```python
from build123d import *

# Parameters (mm, degrees)
F1_DEPTH  = 600
F3_DEPTH  = 600.001
F5_DEPTH  = 20
F7_DEPTH  = 20
F8_W      = 20
F8_H      = 278.7190201738
F8_W_2    = 578.8190174103
F9_DEPTH  = 20
F10_W     = 598.5316634178
F10_H     = 254.7840774059
F11_DEPTH = 2017.6951884178


# Not quite as in the source:
# - a feature names something its author has since deleted; it is built from what else it names


with BuildPart() as f1:
    # F0 (on Right) → F1 (new body)
    with BuildSketch(Plane.YZ):
        with BuildLine():
            ThreePointArc((-413.7737442203, 1932.6941884178), (-235.6171133469, 874.7152717166), (-858.6646769196, 1.2904570733))
            Line((-858.6646769196, 1.2904570733), (841.3353230804, 1.2904570733))
            ThreePointArc((841.3353230804, 1.2904570733), (218.2877610308, 874.7152723164), (396.4443930804, 1932.6941884178))
            Line((396.4443930804, 1932.6941884178), (396.4443930804, 2017.6941884178))
            ThreePointArc((396.4443930804, 2017.6941884178), (199.7456261802, 1948.7680536266), (-8.6646769196, 1951.2904570733))
            ThreePointArc((-8.6646769196, 1951.2904570733), (-217.0749786293, 1948.7680541113), (-413.7737442203, 2017.6941884178))
            Line((-413.7737442203, 2017.6941884178), (-413.7737442203, 1932.6941884178))
        make_face()
    extrude(amount=F1_DEPTH)

    # F2 (on face) → F3 (cut, through all)
    with BuildSketch(Plane.YZ.offset(600)):
        with BuildLine():
            Line((396.4443930804, 2017.6941884178), (-413.7737442203, 2017.6941884178))
            ThreePointArc((-413.7737442203, 2017.6941884178), (-345.7057427079, 1986.5957603046), (-275.2746839195, 1961.3008790249))
            ThreePointArc((-275.2746839195, 1961.3008790249), (-142.5331399832, 1941.2889121961), (-8.6646769196, 1951.2904570733))
            ThreePointArc((-8.6646769196, 1951.2904570733), (125.2037851776, 1941.2889117025), (257.9453283126, 1961.3008776288))
            ThreePointArc((257.9453283126, 1961.3008776288), (328.3763894007, 1986.5957594221), (396.4443930804, 2017.6941884178))
        make_face()
        with BuildLine():
            ThreePointArc((-8.6646769196, 1951.2904570733), (-142.5331399832, 1941.2889121961), (-275.2746839195, 1961.3008790249))
            ThreePointArc((-275.2746839195, 1961.3008790249), (-8.66467791, 1920.6086514411), (257.9453283126, 1961.3008776288))
            ThreePointArc((257.9453283126, 1961.3008776288), (125.2037851776, 1941.2889117025), (-8.6646769196, 1951.2904570733))
        make_face()
    extrude(amount=-F3_DEPTH, mode=Mode.SUBTRACT)

    # F4 (on face) → F5 (join)
    with BuildSketch(Plane.YZ.offset(600)):
        with BuildLine():
            ThreePointArc((-487.8719790556, 1039.6971702576), (-533.5033840935, 470.5867589871), (-858.6646769196, 1.2904570733))
            ThreePointArc((-858.6646769196, 1.2904570733), (-413.6127871917, 445.5030116798), (-207.8719790556, 1039.6971702576))
            Line((-207.8719790556, 1039.6971702576), (-487.8719790556, 1039.6971702576))
        make_face()
        with BuildLine():
            ThreePointArc((190.5426270267, 1039.6971702576), (396.283434362, 445.5030119538), (841.3353230804, 1.2904570733))
            ThreePointArc((841.3353230804, 1.2904570733), (516.1740306428, 470.5867590462), (470.5426270267, 1039.6971702576))
            Line((470.5426270267, 1039.6971702576), (190.5426270267, 1039.6971702576))
        make_face()
    extrude(amount=-F5_DEPTH)

    # F6 (on face) → F7 (join)
    with BuildSketch(Plane(origin=(0, 0, 0), x_dir=(0, -1, 0), z_dir=(-1, 0, 0))):
        with BuildLine():
            ThreePointArc((-841.3353230804, 1.2904570733), (-396.5475396439, 445.0817710452), (-190.6490020093, 1038.7085012816))
            Line((-190.6490020093, 1038.7085012816), (-470.6490020093, 1038.7085012816))
            ThreePointArc((-470.6490020093, 1038.7085012816), (-519.6815928842, 471.2934981386), (-841.3353230804, 1.2904570733))
        make_face()
        with BuildLine():
            ThreePointArc((207.878498719, 1039.6363848164), (413.6290200403, 445.4771111279), (858.6646769196, 1.2904570733))
            ThreePointArc((858.6646769196, 1.2904570733), (536.7100272294, 471.698228356), (487.878498719, 1039.6363848164))
            Line((487.878498719, 1039.6363848164), (207.878498719, 1039.6363848164))
        make_face()
    extrude(amount=-F7_DEPTH)

    # F8 (on face) → F9 (join)
    with BuildSketch(Plane.XY.offset(1039.6363848164)):
        with Locations((10, -348.5189886321)):
            Rectangle(F8_W, F8_H)
        with Locations((309.4095087051, -348.5189886321)):
            Rectangle(F8_W_2, F8_H)
    extrude(amount=F9_DEPTH)

    # F10 (on Top) → F11 (cut, through all)
    with BuildSketch(Plane.XY):
        Polygon((0, 963.8522267342), (0, 254.7840774059), (598.5316634178, 254.7840774059), (598.5316634178, 0), (664.8825407028, 0), (664.8825407028, 963.8522267342), align=None)
        Polygon((-87.8282785416, 0), (0, 0), (0, 254.7840774059), (0, 963.8522267342), (-87.8282785416, 963.8522267342), align=None)
        with Locations((299.2658317089, 127.392038703)):
            Rectangle(F10_W, F10_H)
    extrude(amount=F11_DEPTH, mode=Mode.SUBTRACT)


solid = f1.part
```
Geometry: final body of the model. Coordinates: model frame, mm. A direction names the side the tool comes from. Coordinates: 2 decimals unless noted, no trailing zeros. Loops run counter-clockwise (first coordinate to the right, second up) from the corner with the lowest first, then second, coordinate; pieces in that order, holes last. Notation, with made-up numbers: (-19, 36) -> (40, 36) arc R17 ccw to (40, 65) -> close; hole circle Ø1 at (-17.75, -13). An arc over 180 degrees is marked (long way). Use a Markdown table: item, result. Add a question column.
(1) Access query for faces 1 (the cylindrical face through (590.14, -530.812, 478.212)), 2 (the flat face through (296, -413.774, 1976)), 3 (the cylindrical face through (295.8, -345.316, 1984.771)), 4 (the flat face through (296, 0, 948)), 5 (the flat face through (580, -414, 677)). Directions: +Z, -Z, +X, -X, +Y, -Y. A direction counts if a zero-diameter tool reaches every point of the face in a straight line with its end or side. Return the directions, or none.
(2) Section query D-D, the plane y = -793.5. Return loops of the section in (x, z), plus the area to 3 significant figures.
(3) Section query B-B, the plane y = -375. Return loops of the section in (x, z).
(4) Mould query, pull axis Z, two halves, no side actions, for faces 6 (the flat face through (295, -347, 1059.636)), 7 (the cylindrical face through (9.86, -539.45, 464.11)), 8 (the flat face through (296, -435, 1.29)), 9 (the flat face through (600, -245, 800)). Classes: pulls with the +Z half, pulls with the -Z half, needs draft (parallel to the pull), parting line crosses it, or undercut.
(5) Pin query (flat end, axial travel): pin 1 Ø1 at (x, z) = (103, 516) entering from -Y; pin 2 Ø22 at (x, y) = (590, -332) entering from +Z; pin 3 Ø10 at (y, z) = (-303, 1049.5) entering from +X. Return the tip coordinate at first contact, or that it passes through.
(6) Line query: line 1 along Z through (x, y) = (159, -365.5); line 2 along Z through (x, y) = (300, -457); line 3 along Y through (x, z) = (259, 1554.5). Output: solid intervals per line, ascending.
(7) Section query C-C, the plane z = 634.5. Return loops of the section in (x, y).
(8) Section query A-A, the plane x = 338. Return loops of the section in (y, z).
Answer:
| question | item | result |
|---|---|---|
| 1 | face 1 | +X, -Y |
| 1 | face 2 | +Z, +X, -X, -Y |
| 1 | face 3 | +Z, +X, -X, +Y |
| 1 | face 4 | +Z, -Z, +X, -X, +Y |
| 1 | face 5 | -Y |
| 2 | outline | (0, 1.29) -> (600, 1.29) -> (600, 61.05) -> (580, 61.05) -> (580, 44.53) -> (20, 44.53) -> (20, 62.4) -> (0, 62.4) -> close |
| 2 | area | 26,600 mm^2 |
| 3 | outline | (0, 1.29) -> (600, 1.29) -> (600, 1039.7) -> (598.82, 1039.7) -> (598.82, 1059.64) -> (0, 1059.64) -> close; (0, 1866.94) -> (600, 1866.94) -> (600, 1997.74) -> (0, 1997.74) -> close; hole (20, 511) -> (580, 511) -> (580, 1039.64) -> (20, 1039.64) -> close |
| 4 | face 6 | undercut |
| 4 | face 7 | undercut |
| 4 | face 8 | pulls with the -Z half |
| 4 | face 9 | needs draft |
| 5 | pin 1 | stops at y = -372.52 |
| 5 | pin 2 | stops at z = 1983.84 |
| 5 | pin 3 | stops at x = 598.82 |
| 6 | line 1 | z = 1.29 to 528.46, 1039.64 to 1059.64, 1849.48 to 1993.38 |
| 6 | line 2 | z = 1.29 to 380.39, 1039.64 to 1059.64 |
| 6 | line 3 | y = -248.45 to 0 |
| 7 | outline | (0, -492.08) -> (20, -492.08) -> (20, -314.37) -> (580, -314.37) -> (580, -488.92) -> (600, -488.92) -> (600, 0) -> (0, 0) -> close |
| 8 | outline | (-858.66, 1.29) -> (0, 1.29) -> (0, 1920.65) arc R893.74 cw to (-275.27, 1961.3) arc R600 cw to (-413.77, 2017.69) -> (-413.77, 1932.69) arc R1400 cw to start; (-487.88, 1039.64) -> (-209.16, 1039.64) -> (-209.16, 1059.64) -> (-487.88, 1059.64) -> close |
